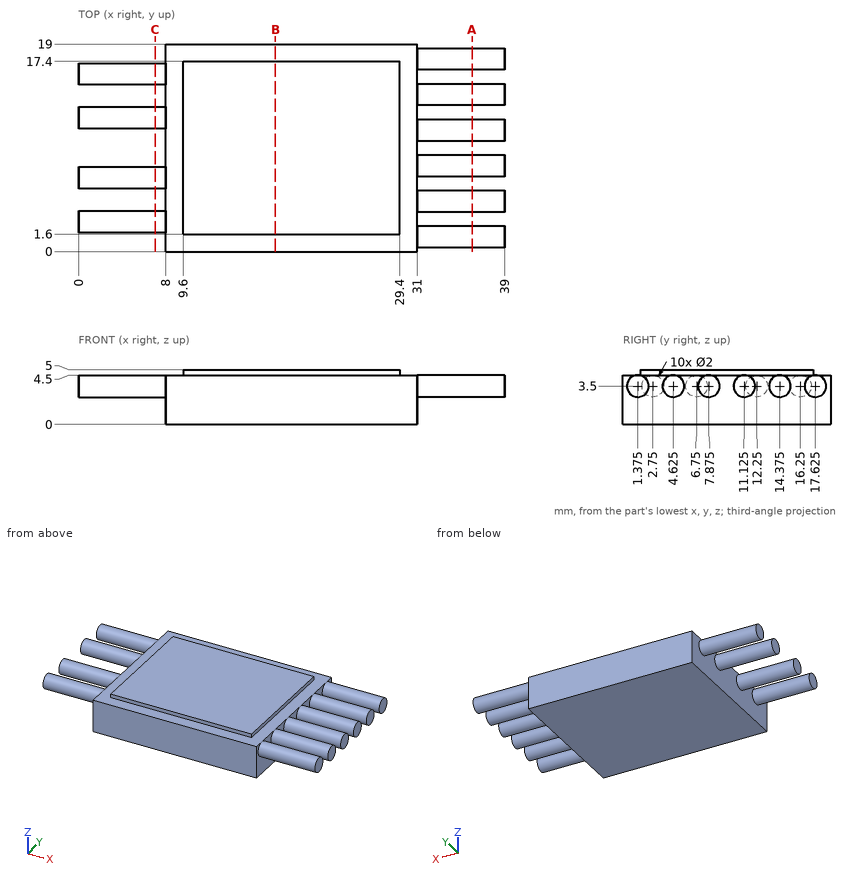
Study the drawing (mm; zero at the part's minimum x, y, z) and answer. Coordinates: 2 decimals unless noted, no trailing zeros. Write each loop counter-clockwise with the first axis right and the second up, starting at its lowest first coordinate (ties: lowest second). Pieces come first, ordered by that corner, then holes. Notation, with made-up numbers: (54, 4.5) - (79, 4.5) arc R25 ccw to (79, 41.5) - close; hole circle Ø6 at (31.5, -33.5). An arc over 180 degrees is marked (long way). Return JSON: item names as keys, results as strings. Group by question number.
1. A cutting plane is placed at C-C, the plane x = 7. Determine the outline of the cut face in (y, z).
2. Straight lines are drawn through the part: L1, parallel to X at y = 7, z = 4.1; L2, parallel to X at y = 8.5, z = 3.55; L3, parallel to Z at x = 30.5, y = 2.25. For each, find the intervals that lie inside material, in ascending order.
3. Given pin 1 (1.3 mm diameter, centred on y = 8, z = 1.5, fed in from +X), flat-ended and moving along its own axis, determine where the tip first touches the part or whether it passes through.
4. A cutting plane is placed at B-B, the plane x = 18. Determine the outline of the cut face in (y, z), plus the area to 3 significant figures.
5. A cutting plane is placed at A-A, the plane x = 36. Determine the outline of the cut face in (y, z) (3 decimals), plus the area to 3 significant figures.
Ans:
{
 "1": {"outline": "circle Ø2 at (2.75, 3.5); circle Ø2 at (6.75, 3.5); circle Ø2 at (12.25, 3.5); circle Ø2 at (16.25, 3.5)"},
 "2": {"L1": "0 to 31", "L2": "8 to 39", "L3": "0 to 4.5"},
 "3": {"pin 1": "x = 31"},
 "4": {"outline": "(0, 0) - (19, 0) - (19, 4.5) - (17.4, 4.5) - (17.4, 5) - (1.6, 5) - (1.6, 4.5) - (0, 4.5) - close", "area": "93.4 mm²"},
 "5": {"outline": "circle Ø2 at (1.375, 3.5); circle Ø2 at (4.625, 3.5); circle Ø2 at (7.875, 3.5); circle Ø2 at (11.125, 3.5); circle Ø2 at (14.375, 3.5); circle Ø2 at (17.625, 3.5)", "area": "18.8 mm²"}
}
